Input: part model. Units: mm. Frame: model coordinates. A direction names the side the tool comes from. Give positions to 0.01 mm unless a question says otherwise; leave off trailing zeros. Write each loop counter-clockwise with the first axis right and the second up, starting at its lowest first coordinate (ties: lowest second). Pieces come first, ordered by that corner, then holes. Notation, with made-up numbers: M -15,-13 L 41,-13 A10 ccw 41,-6 Z; hole C -31,89.5 d10. An arc over 180 degrees is marked long. Use CSV: the item, a comma, the result in double quotes. Start each with the question number.
from build123d import *

# Parameters (mm, degrees)
PAD_DEPTH            = 238.75
SKETCH001_R          = 18
POCKET_DEPTH         = 6
BODY_ROLL_ANGLE      = 180
BODY_PLACEMENT_ANGLE = 90


with BuildPart() as part:
    # Sketch → Pad (new body)
    with BuildSketch(Plane.XY):
        Polygon((0, 50), (0, 0), (50, 0), (50, 6), (6, 6), (6, 50), align=None)
    pad = extrude(amount=PAD_DEPTH)

    # Mirrored: Pad across face of Pad
    add(pad.mirror(Plane(origin=(3, 50, 119.375), x_dir=(-1, 0, 0), z_dir=(0, 1, 0))))

    # Sketch001 (on Face5 of Pad) → Pocket (cut)
    with BuildSketch(Plane.YZ.offset(6)):
        with Locations((50, 71.25)):
            Circle(SKETCH001_R)
    extrude(amount=-POCKET_DEPTH, mode=Mode.SUBTRACT)


with BuildPart() as part_1:
    # Body roll: moved
    add(part.part.rotate(Axis((0, 0, 0), (1, 0, 0)), BODY_ROLL_ANGLE))


with BuildPart() as part_2:
    # Body placement: moved
    add(part_1.part.moved(Location((-50, 0, 238.75))).rotate(Axis((-50, 0, 238.75), (0, 0, 1)), BODY_PLACEMENT_ANGLE))


solid = part_2.part
Q1. Pull-direction query (X, two-part tool) for faces 3 (the flat face through (-1, 0, 121)), 4 (the cylindrical face through (8.306, 3.042, 183.469)), 5 (the flat face through (-44, 28, 121)), 6 (the flat face through (50, 25, 121)); classes: released by +X, released by -X, zero draft, split by the parting line, or undercut.
Q2. Set-up query: faces 1 (the flat face through (-47, 50, 121)), 2 (the flat face through (44, 28, 121)). Return all of +Z, -Z, +X, -X, +Y, -Y with unobstructed straight access to the full face (end or side cutting, diameter ignored); none if empty.
Q3. Section C-C, the plane y = 45. Return the cut outline in (x, z).
Q4. First-contact query: pin 1 Ø1.5 at (x, z) = (-24.5, 204.5) entering from +Y. Flat tip, straight axial feed; report the tip coordinate or a pass-through.
Q5. Material intervals for L1, parallel to X at y = 7.5, z = 226; L2, parallel to X at y = 2, z = 167.5; L3, parallel to Z at x = 0, y = 1.5, sorted ascending. Write a range as [from, to].
Q6. Section D-D, the plane z = 210.5. Return the cut outline in (x, y), and give its area (3 significant figures).
Q7. Section B-B, the plane z = 167.5. Return the cut outline in (x, y).
Q8. Section A-A, the plane x = 0. Return the cut outline in (y, z).
Check result:
1,face 3,"zero draft"
1,face 4,"undercut"
1,face 5,"undercut"
1,face 6,"released by +X"
2,face 1,"+Z, -Z, +X, -X, +Y"
2,face 2,"+Z, -Z, +Y"
3,outline,"M -50,0 L -44,0 L -44,238.75 L -50,238.75 Z; M 44,0 L 50,0 L 50,238.75 L 44,238.75 Z"
4,pin 1,"stops at y = 6"
5,L1,"x = [-50, -44], [44, 50]"
5,L2,"x = [-50, -18], [18, 50]"
5,L3,"z = [0, 149.5], [185.5, 238.75]"
6,outline,"M -50,0 L 50,0 L 50,50 L 44,50 L 44,6 L -44,6 L -44,50 L -50,50 Z"
6,area,"1,130 mm²"
7,outline,"M -50,0 L -18,0 L -18,6 L -44,6 L -44,50 L -50,50 Z; M 18,0 L 50,0 L 50,50 L 44,50 L 44,6 L 18,6 Z"
8,outline,"M 0,0 L 6,0 L 6,149.5 L 0,149.5 Z; M 0,185.5 L 6,185.5 L 6,238.75 L 0,238.75 Z"
